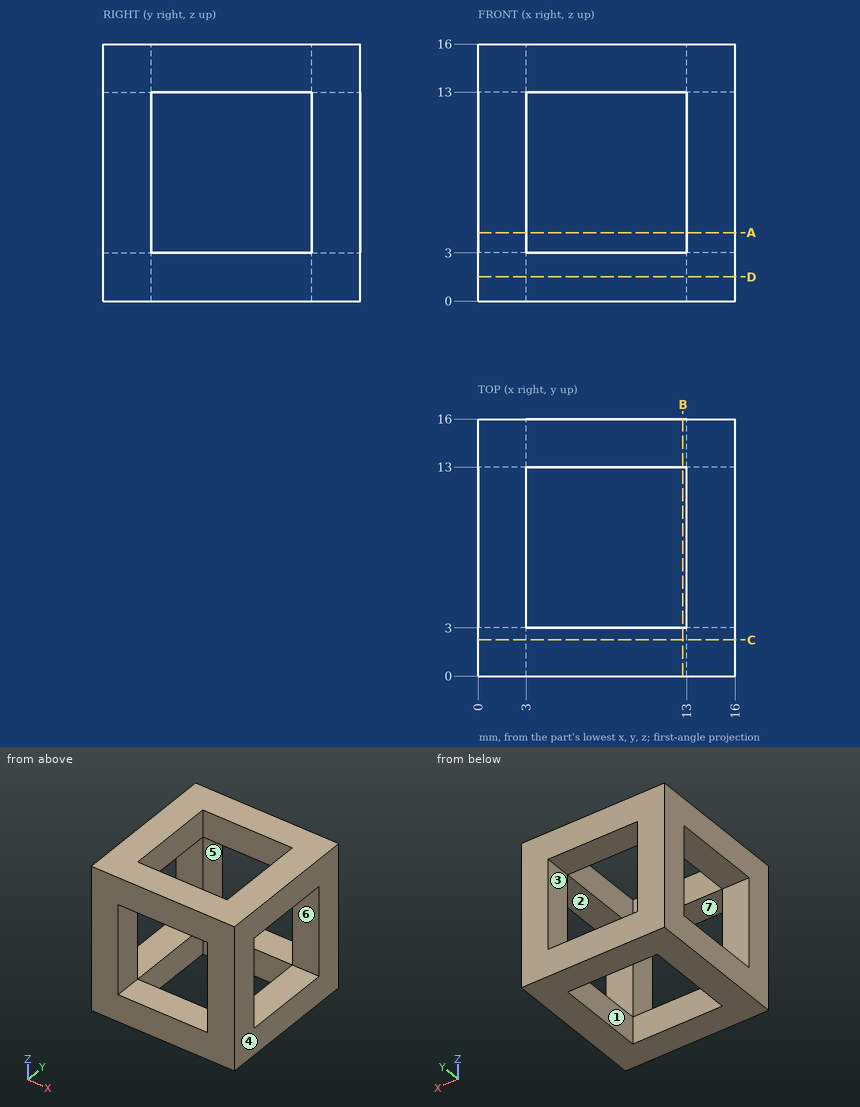
Geometry check sheet. Reference: drawing and pictorial views, mm from the part's lowest x, y, z. A direction names the side the tool comes from. Round coordinates to 2 decimals unless told otherwise and drop trailing zeros. Order: outer loops, then holes, each group sorted by start corner. A loop starts at its lowest first (then second) coordinate and runs counter-clockwise, first axis right, second up. Notation, with made-up numbers: (9.5, 46) - (24.5, 46) arc R19 ccw to (24.5, 70) - close; hole circle Ø7 at (-0.5, -12). An arc over 180 degrees is marked (long way). One line per question, with ' | ' between items. Start each with the question number.
(1) Thickness scan on L1, parallel to Z at x = 1.5, y = 6.75. Record the ranges inside material, lowest first. Write a range as [from, to].
(2) Sectioned sample at C-C on y = 2.25. Record the cut outline in (x, z), and give its area (3 significant figures).
(3) Sectioned sample at A-A on z = 4.25. Record the cut outline in (x, y).
(4) Release check for a two-part mould opening along X. For the marked faces 4, 5, 6 and 7 record: released by +X, released by -X, zero draft, split by the parting line, or undercut.
(5) Access from +Z, -Z, +X, -X, +Y, -Y to the whole of each face (thin tool, end or side, straight path). Record for the marked faces 1, 2 and 3.
Conclusion:
1) L1: z = [0, 3], [13, 16]
2) outline: (0, 0) - (16, 0) - (16, 16) - (0, 16) - close; hole (3, 3) - (13, 3) - (13, 13) - (3, 13) - close | area: 156 mm2
3) outline: (0, 0) - (3, 0) - (3, 3) - (0, 3) - close; (0, 13) - (3, 13) - (3, 16) - (0, 16) - close; (13, 0) - (16, 0) - (16, 3) - (13, 3) - close; (13, 13) - (16, 13) - (16, 16) - (13, 16) - close
4) face 4: released by +X | face 5: undercut | face 6: zero draft | face 7: undercut
5) face 1: +Z, -Z | face 2: +X, -X | face 3: +Y, -Y
